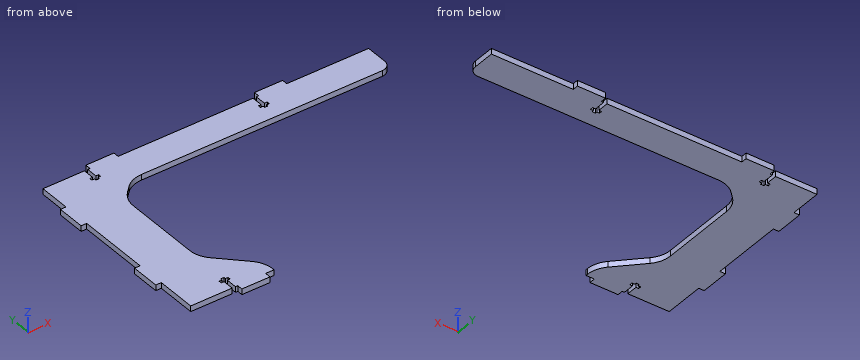
from build123d import *

# Parameters (mm, degrees)
BOSS_EXTRUDE1_DEPTH = 5.08


with BuildPart() as part:
    # Sketch1 → Boss-Extrude1 (new body)
    with BuildSketch(Plane.XY):
        with BuildLine():
            Line((-114.376804032, 88.667051475), (-139.776804032, 88.667051475))
            Line((-139.776804032, 88.667051475), (-139.776804032, 93.747051475))
            Line((-139.776804032, 93.747051475), (-141.822276948, 93.747051475))
            Line((-141.822276948, 93.747051475), (-141.822276948, 103.713000769))
            Line((-141.822276948, 103.713000769), (-139.282276948, 103.713000769))
            Line((-139.282276948, 103.713000769), (-139.282276948, 106.213000769))
            Line((-139.282276948, 106.213000769), (-141.822276948, 106.213000769))
            Line((-141.822276948, 106.213000769), (-141.822276948, 107.947051475))
            Line((-141.822276948, 107.947051475), (-144.822276948, 107.947051475))
            Line((-144.822276948, 107.947051475), (-144.822276948, 106.213000769))
            Line((-144.822276948, 106.213000769), (-147.362276948, 106.213000769))
            Line((-147.362276948, 106.213000769), (-147.362276948, 103.713000769))
            Line((-147.362276948, 103.713000769), (-144.822276948, 103.713000769))
            Line((-144.822276948, 103.713000769), (-144.822276948, 93.747051475))
            Line((-144.822276948, 93.747051475), (-182.269486813, 93.747051475))
            Line((-182.269486813, 93.747051475), (-182.269486813, 129.81075177))
            Line((-182.269486813, 129.81075177), (-187.286518352, 129.81075177))
            Line((-187.286518352, 129.81075177), (-187.286518352, 155.871504364))
            Line((-187.286518352, 155.871504364), (-182.269486813, 155.871504364))
            Line((-182.269486813, 155.871504364), (-182.269486813, 212.837023738))
            Line((-182.269486813, 212.837023738), (-182.269486813, 221.371776332))
            Line((-182.269486813, 221.371776332), (-187.286518352, 221.371776332))
            Line((-187.286518352, 221.371776332), (-187.286518352, 246.771776332))
            Line((-187.286518352, 246.771776332), (-182.269486813, 246.771776332))
            Line((-182.269486813, 246.771776332), (-182.269486813, 274.961476627))
            Line((-182.269486813, 274.961476627), (-144.822276948, 274.961476627))
            Line((-144.822276948, 274.961476627), (-144.822276948, 264.995527332))
            Line((-144.822276948, 264.995527332), (-147.362276948, 264.995527332))
            Line((-147.362276948, 264.995527332), (-147.362276948, 262.495527332))
            Line((-147.362276948, 262.495527332), (-144.822276948, 262.495527332))
            Line((-144.822276948, 262.495527332), (-144.822276948, 260.761476627))
            Line((-144.822276948, 260.761476627), (-141.822276948, 260.761476627))
            Line((-141.822276948, 260.761476627), (-141.822276948, 262.495527332))
            Line((-141.822276948, 262.495527332), (-139.282276948, 262.495527332))
            Line((-139.282276948, 262.495527332), (-139.282276948, 264.995527332))
            Line((-139.282276948, 264.995527332), (-141.822276948, 264.995527332))
            Line((-141.822276948, 264.995527332), (-141.822276948, 274.961476627))
            Line((-141.822276948, 274.961476627), (-139.776804032, 274.961476627))
            Line((-139.776804032, 274.961476627), (-139.776804032, 280.041476627))
            Line((-139.776804032, 280.041476627), (-114.376804032, 280.041476627))
            Line((-114.376804032, 280.041476627), (-114.376804032, 274.961476627))
            Line((-114.376804032, 274.961476627), (-106.810604162, 274.961476627))
            Line((-106.810604162, 274.961476627), (7.577723052, 274.961476627))
            Line((7.577723052, 274.961476627), (7.577723052, 264.995527332))
            Line((7.577723052, 264.995527332), (5.037723052, 264.995527332))
            Line((5.037723052, 264.995527332), (5.037723052, 262.495527332))
            Line((5.037723052, 262.495527332), (7.577723052, 262.495527332))
            Line((7.577723052, 262.495527332), (7.577723052, 260.761476627))
            Line((7.577723052, 260.761476627), (10.577723052, 260.761476627))
            Line((10.577723052, 260.761476627), (10.577723052, 262.495527332))
            Line((10.577723052, 262.495527332), (13.117723052, 262.495527332))
            Line((13.117723052, 262.495527332), (13.117723052, 264.995527332))
            Line((13.117723052, 264.995527332), (10.577723052, 264.995527332))
            Line((10.577723052, 264.995527332), (10.577723052, 274.961476627))
            Line((10.577723052, 274.961476627), (12.623195968, 274.961476627))
            Line((12.623195968, 274.961476627), (12.623195968, 280.041476627))
            Line((12.623195968, 280.041476627), (38.023195968, 280.041476627))
            Line((38.023195968, 280.041476627), (38.023195968, 274.961476627))
            Line((38.023195968, 274.961476627), (112.050844633, 274.961476627))
            Line((112.050844633, 274.961476627), (112.050844633, 255.184968454))
            ThreePointArc((112.050844633, 255.184968454), (109.586677712, 249.235943253), (103.63765251, 246.771776332))
            Line((103.63765251, 246.771776332), (-114.102022694, 246.771776332))
            ThreePointArc((-114.102022694, 246.771776332), (-122.850165958, 245.031662445), (-130.266483712, 240.076237349))
            Line((-130.266483712, 240.076237349), (-135.253616385, 235.089104676))
            ThreePointArc((-135.253616385, 235.089104676), (-140.20904148, 227.672786922), (-141.949155367, 218.924643658))
            Line((-141.949155367, 218.924643658), (-141.949155367, 149.783884443))
            ThreePointArc((-141.949155367, 149.783884443), (-140.20904148, 141.035741179), (-135.253616385, 133.619423425))
            Line((-135.253616385, 133.619423425), (-113.506143144, 111.871950184))
            ThreePointArc((-113.506143144, 111.871950184), (-108.550718048, 104.45563243), (-106.810604162, 95.707489166))
            Line((-106.810604162, 95.707489166), (-106.810604162, 93.993771805))
            Line((-106.810604162, 93.993771805), (-114.376804032, 93.993771805))
            Line((-114.376804032, 93.993771805), (-114.376804032, 88.93863086))
            Line((-114.376804032, 88.93863086), (-114.376804032, 88.667051475))
        make_face()
    extrude(amount=BOSS_EXTRUDE1_DEPTH)


solid = part.part
The listing builds one solid part. Answer for the finished solid, in the listing's coordinates (mm). Round coordinates to 2 decimals unless told otherwise and drop trailing zeros. Write each loop counter-clockwise with the first axis right and the second up, starting at its lowest first coordinate (ties: lowest second). Pieces come first, ordered by that corner, then holes. Notation, with made-up numbers: M 14,-7 L 48,-7 A22 ccw 48,4 Z; hole C 59.25,86.25 d9. An arc over 180 degrees is marked long. Write each question's results on one line, items separated by ' | '. Start each with the question number.
Item 1: Straight lines are drawn through the part: L1, parallel to X at y = 261, z = 4.45; L2, parallel to X at y = 203.5, z = 4; L3, parallel to X at y = 150, z = 0.8. For each, find the intervals that lie inside material, in ascending order. Write a range as [from, to].
Item 2: A cutting plane is placed at A-A on x = -125.5. Write down the section's boundary in (y, z).
Item 3: Flat-ended cylindrical pins translate along their axes: pin 1 Ø1.5 at (y, z) = (90.5, 3) entering from +X; pin 2 Ø1.2 at (y, z) = (104.5, 2.5) entering from -X; pin 3 Ø2 at (x, z) = (15, 2) entering from -Y. Find the tip coordinate at first contact, or state that the pin passes through.
Item 4: A cutting plane is placed at C-C on y = 182. Write down the section's boundary in (x, z), and give its area (3 significant figures).
Item 5: A cutting plane is placed at B-B on x = -155.5. Write down the section's boundary in (y, z), and give its area (3 significant figures).
Check sheet entries:
1) L1: [-182.27, -144.82], [-141.82, 7.58], [10.58, 112.05] | L2: [-182.27, -141.95] | L3: [-187.29, -141.95]
2) outline: M 88.67,0 L 123.87,0 L 123.87,5.08 L 88.67,5.08 Z; M 243.73,0 L 280.04,0 L 280.04,5.08 L 243.73,5.08 Z
3) pin 1: x = -114.38 | pin 2: x = -182.27 | pin 3: y = 246.77
4) outline: M -182.27,0 L -141.95,0 L -141.95,5.08 L -182.27,5.08 Z | area: 205 mm²
5) outline: M 93.75,0 L 274.96,0 L 274.96,5.08 L 93.75,5.08 Z | area: 921 mm²
